The model under review builds one solid part; all positions refer to its coordinate system, in mm. A direction names the side the tool comes from. Coordinates: 2 decimals unless noted, no trailing zeros. Write each loop counter-clockwise with the first axis right and the second up, starting at its lowest first coordinate (ties: lowest second). Pieces come first, ordered by that corner, then holes. Notation, with made-up numbers: (45, 47) - (88, 47) arc R21 cw to (88, 59) - close; hole circle Ø1 at (-38.5, 58.5). An arc over 180 degrees is marked (long way). Return JSON: item names as keys, results as strings. Group by question number.
(1) To check wall thickness, follow L1, parallel to X at y = 3, z = 4.2; L2, parallel to X at y = -18, z = 0.55; L3, parallel to Y at x = 37.5, z = 2.55. State the ranges of each line that lie inside material, in increasing order. Write a range as from..to.
(2) We need section B-B on x = 67. State the section outline as (y, z) points, then the cut area to 3 significant figures.
(3) Tool access review of faces 1 (the face through (21, 26.707, 3)), 2 (the face through (0, -41.879, 2)), 3 (the face through (-33.789, 49, 3)), 4 (the face through (121, -30.846, 2)): name each direction out of +Z, -Z, +X, -X, +Y, -Y from which nothing blocks a thin tool from reaching the whole face with its end or side.
(4) We need section D-D on z = 2.95. Give the number of separate pieces and of enclosed holes in the cut face, then the cut area to 3 significant figures.
(5) We need section A-A on y = -14. State the section outline as (x, z) points.
(6) Draft analysis for pull direction X (two halves, no side actions). For faces 5 (the face through (-52.415, -73.072, 2.465)), 6 (the face through (98, 47.327, 3)), 7 (the face through (-79.116, 68, 3)), 8 (the face through (80.308, 68, 3)), state which applies: released by +X, released by -X, zero draft, split by the parting line, or undercut.
(7) We need section C-C on y = -45. State the section outline as (x, z) points, then the cut area to 3 significant figures.
(8) For pin 1 Ø1.5 at (x, z) = (22.5, 1.5) entering from -Y; pin 2 Ø2.5 at (x, y) = (-5.42, -5.67) entering from +Z; pin 3 Ø5 at (x, y) = (6.61, 29.33) entering from +Z; pin 4 Ø2.5 at (y, z) = (-6, 2) entering from +X, all flat-tipped, find the tip position at first contact; note any pin that passes through.
```python
from build123d import *

# Parameters (mm, degrees)
SKETCH1_R           = 2
SKETCH1_W           = 33.838048367
SKETCH1_H           = 82.031632405
BOSS_EXTRUDE1_DEPTH = 5
SKETCH6_W           = 26.358753283
SKETCH6_H           = 29.759882739
CUT_EXTRUDE5_DEPTH  = 10
CUT_EXTRUDE7_DEPTH  = 10
SKETCH8_R           = 110
CUT_EXTRUDE8_DEPTH  = 10
SKETCH9_W           = 34.735720487
SKETCH9_H           = 8.029761027
BOSS_EXTRUDE2_DEPTH = 5
SKETCH10_W          = 47.255249557
SKETCH10_H          = 69.524861462
SKETCH10_W_2        = 47.255249556
CUT_EXTRUDE9_DEPTH  = 10


with BuildPart() as part:
    # Sketch1 → Boss-Extrude1 (new body)
    with BuildSketch(Plane.XY):
        with BuildLine():
            Line((-67.377293169, 102.297329585), (-124.936746461, 102.297329585))
            Line((-124.936746461, 102.297329585), (-124.953483971, 82.555494847))
            Line((-124.953483971, 82.555494847), (-124.958588565, 69.121872443))
            Line((-124.958588565, 69.121872443), (-124.95889847, 54.500614803))
            Line((-124.95889847, 54.500614803), (-115.116370276, 54.500614803))
            Line((-115.116370276, 54.500614803), (-115.116370276, -30.846433579))
            Line((-115.116370276, -30.846433579), (-124.960166164, -30.846433579))
            Line((-124.960166164, -30.846433579), (-124.960166164, -103.402915432))
            Line((-124.960166164, -103.402915432), (-69.927203874, -103.402915432))
            Line((-69.927203874, -103.402915432), (-34.406465086, -41.879191129))
            Line((-34.406465086, -41.879191129), (35.597608304, -41.879191129))
            Line((35.597608304, -41.879191129), (71.118347092, -103.402915432))
            Line((71.118347092, -103.402915432), (126.151309382, -103.402915432))
            Line((126.151309382, -103.402915432), (126.151309382, -30.846433579))
            Line((126.151309382, -30.846433579), (116.434490518, -30.846433579))
            ThreePointArc((116.434490518, -30.846433579), (116.344704203, -30.80924287), (116.307513493, -30.719456554))
            Line((116.307513493, -30.719456554), (116.307513493, 54.373637777))
            ThreePointArc((116.307513493, 54.373637777), (116.344704203, 54.463424093), (116.434490518, 54.500614803))
            Line((116.434490518, 54.500614803), (126.150041687, 54.500614803))
            Line((126.150041687, 54.500614803), (126.149731996, 69.11181019))
            Line((126.149731996, 69.11181019), (126.144618663, 82.565551548))
            Line((126.144618663, 82.565551548), (126.127889679, 102.297329585))
            Line((126.127889679, 102.297329585), (68.568436387, 102.297329585))
            ThreePointArc((68.568436387, 102.297329585), (0.595571609, 72.327090612), (-67.377293169, 102.297329585))
        make_face()
        with Locations((-5.420244594, -5.672909388)):
            Circle(SKETCH1_R, mode=Mode.SUBTRACT)
        with Locations((-36.420244594, -5.672909388)):
            Circle(SKETCH1_R, mode=Mode.SUBTRACT)
        with Locations((-36.420244594, 29.327090612)):
            Circle(SKETCH1_R, mode=Mode.SUBTRACT)
        with Locations((-5.420244594, 29.327090612)):
            Circle(SKETCH1_R, mode=Mode.SUBTRACT)
        with Locations((6.611387811, 29.327090612)):
            Circle(SKETCH1_R, mode=Mode.SUBTRACT)
        with Locations((6.611387811, -5.672909388)):
            Circle(SKETCH1_R, mode=Mode.SUBTRACT)
        with Locations((37.611387811, -5.672909388)):
            Circle(SKETCH1_R, mode=Mode.SUBTRACT)
        with Locations((37.611387811, 29.327090612)):
            Circle(SKETCH1_R, mode=Mode.SUBTRACT)
        with Locations((58.530411994, 11.827090612)):
            Rectangle(SKETCH1_W, SKETCH1_H, mode=Mode.SUBTRACT)
        with Locations((-57.339268778, 11.827090612)):
            Rectangle(SKETCH1_W, SKETCH1_H, mode=Mode.SUBTRACT)
    extrude(amount=BOSS_EXTRUDE1_DEPTH)

    # Sketch6 → Cut-Extrude5 (cut)
    with BuildSketch(Plane.XY.offset(5)):
        with Locations((-20.920244594, 11.827090611)):
            Rectangle(SKETCH6_W, SKETCH6_H)
        with Locations((20.920244594, 11.827090611)):
            Rectangle(SKETCH6_W, SKETCH6_H)
    extrude(amount=-CUT_EXTRUDE5_DEPTH, mode=Mode.SUBTRACT)

    # Sketch7 → Cut-Extrude7 (cut)
    with BuildSketch(Plane.XY.offset(5)):
        Polygon((36.611387811, 79.275951145), (36.611387811, 38.327090612), (-33.788939324, 38.327090612), (-33.788939324, 77.421207896), (-33.788939324, 95.121170758), (36.611387811, 95.121170758), align=None)
    extrude(amount=-CUT_EXTRUDE7_DEPTH, mode=Mode.SUBTRACT)

    # Sketch8 → Cut-Extrude8 (cut)
    with BuildSketch(Plane(origin=(0, 0, 0), x_dir=(-1, 0, 0), z_dir=(0, 0, -1))):
        with Locations((-0.595571609, 164.393850159)):
            Circle(SKETCH8_R)
    extrude(amount=-CUT_EXTRUDE8_DEPTH, mode=Mode.SUBTRACT)

    # Sketch9 → Boss-Extrude2 (add)
    with BuildSketch(Plane.XY.offset(5)):
        with Locations((-107.568886218, 106.312210099)):
            Rectangle(SKETCH9_W, SKETCH9_H)
        with Locations((108.760029436, 106.312210099)):
            Rectangle(SKETCH9_W, SKETCH9_H)
    extrude(amount=-BOSS_EXTRUDE2_DEPTH)

    # Sketch10 → Cut-Extrude9 (cut)
    with BuildSketch(Plane.XY.offset(5)):
        with Locations((103.935138271, 82.089521343)):
            Rectangle(SKETCH10_W, SKETCH10_H)
        with Locations((-102.743995054, 82.089521343)):
            Rectangle(SKETCH10_W_2, SKETCH10_H)
    extrude(amount=-CUT_EXTRUDE9_DEPTH, mode=Mode.SUBTRACT)


solid = part.part
```
Ans:
{
 "1": {"L1": "-115.12..-74.26, -40.42..-34.1, -7.74..7.74, 34.1..41.61, 75.45..116.31", "L2": "-115.12..-74.26, -40.42..41.61, 75.45..116.31", "L3": "-45.17..-7.67, -3.68..27.33, 31.32..60.77"},
 "2": {"outline": "(-96.27, 0) - (-29.19, 0) - (-29.19, 5) - (-96.27, 5) - close; (52.84, 0) - (76.7, 0) - (76.7, 5) - (52.84, 5) - close", "area": "455 mm²"},
 "3": {"face 1": "+Z, -Z", "face 2": "+Z, -Z, -Y", "face 3": "+Z, -Z, +Y", "face 4": "+Z, -Z, +X, +Y"},
 "4": {"separate pieces": "1", "enclosed holes": "12", "area": "24,100 mm²"},
 "5": {"outline": "(-115.12, 0) - (-74.26, 0) - (-74.26, 5) - (-115.12, 5) - close; (-40.42, 0) - (41.61, 0) - (41.61, 5) - (-40.42, 5) - close; (75.45, 0) - (116.31, 0) - (116.31, 5) - (75.45, 5) - close"},
 "6": {"face 5": "undercut", "face 6": "zero draft", "face 7": "released by -X", "face 8": "released by +X"},
 "7": {"outline": "(-124.96, 0) - (-36.21, 0) - (-36.21, 5) - (-124.96, 5) - close; (37.4, 0) - (126.15, 0) - (126.15, 5) - (37.4, 5) - close", "area": "888 mm²"},
 "8": {"pin 1": "y = -41.88", "pin 2": "through", "pin 3": "z = 5", "pin 4": "x = 116.31"}
}
